Verification items for the finished model (mm, model axes). A direction names the side the tool comes from. Give positions to 0.01 mm unless a question says otherwise; leave off trailing zeros. Order: outer loops, then holes, each group sorted by start corner. A loop starts at its lowest first (then second) coordinate and runs counter-clockwise, first axis right, second up. Notation, with made-up numbers: (5, 61) -> (48, 61) arc R13 cw to (48, 79) -> close; hole circle Ø2 at (16, 29.25). An arc over 180 degrees is marked (long way). Return JSON: item names as keys, results as strings. Group by question number.
(1) Tool access check on faces 1 (the face through (73.74, 16.07, -5.06)), 2 (the face through (9.648, 0.359, 16.406)). Record the directions out of +Z, -Z, +X, -X, +Y, -Y that give a thin tool (end or side, any length) a straight path to the whole face; none if there is none.
(2) Depth check by flat-ended pin: pin 1 Ø6 at (x, y) = (115.5, 7.5) entering from -Z; pin 2 Ø1 at (x, y) = (53, 12) entering from +Z; pin 3 Ø1.5 at (x, z) = (51.5, 8) entering from -Y. Enter the tip coordinate at first touch or a pass-through.
(3) Cross-section at B-B on x = 69. Enter the section's corners in (y, z).
(4) Release check for a two-part mould opening along X. For faces 3 (the face through (75.81, 15.28, -4.81)), 4 (the face through (-0.25, -1.953, -14.877)) record: pulls with the +X half, pulls with the -X half, needs draft (parallel to the pull), parting line crosses it, or undercut.
(5) Cross-section at A-A on z = 0. Enter the section's corners in (x, y).
(6) Thickness scan on line 1 along Y through (x, z) = (79, 0); line 2 along Z through (x, y) = (149.85, 0). Record the ranges inside material, lowest first.
from build123d import *

# Parameters (mm, degrees)
SKETCH2_R          = 1.1938
CUT_EXTRUDE1_DEPTH = 16.84655


with BuildPart() as part:
    # Sketch1 → Revolve1 (revolve)
    with BuildSketch(Plane.XY):
        with BuildLine():
            Line((-0.882617928, 15.379667928), (-0.508, 15.00505))
            Line((-0.508, 15.00505), (0, 15.00505))
            Line((0, 15.00505), (1.016, 16.02105))
            Line((1.016, 16.02105), (148.5392, 16.02105))
            Line((148.5392, 16.02105), (149.5552, 15.00505))
            Line((149.5552, 15.00505), (150.0632, 15.00505))
            Line((150.0632, 15.00505), (150.437817928, 15.379667928))
            ThreePointArc((150.437817928, 15.379667928), (150.475015367, 15.46947049), (150.437817928, 15.559273051))
            Line((150.437817928, 15.559273051), (149.44812049, 16.54897049))
            ThreePointArc((149.44812049, 16.54897049), (149.118506367, 16.769211605), (148.7297, 16.84655))
            Line((148.7297, 16.84655), (0.8255, 16.84655))
            ThreePointArc((0.8255, 16.84655), (0.436693633, 16.769211605), (0.10707951, 16.54897049))
            Line((0.10707951, 16.54897049), (-0.882617928, 15.559273051))
            ThreePointArc((-0.882617928, 15.559273051), (-0.919815367, 15.46947049), (-0.882617928, 15.379667928))
        make_face()
    revolve(axis=Axis((149.5552, 0, 0), (-1, 0, 0)))

    # Sketch2 → Cut-Extrude1 (cut)
    with BuildSketch(Plane.XY):
        with Locations((8.509, 0)):
            Circle(SKETCH2_R)
    extrude(amount=CUT_EXTRUDE1_DEPTH, mode=Mode.SUBTRACT)


solid = part.part
Verdict:
{
 "1": {"face 1": "+X, -X", "face 2": "+Z"},
 "2": {"pin 1": "z = -16.23", "pin 2": "z = 12.31", "pin 3": "y = -15.21"},
 "3": {"outline": "circle Ø33.69 at (0, 0); hole circle Ø32.04 at (0, 0)"},
 "4": {"face 3": "undercut", "face 4": "needs draft"},
 "5": {"outline": "(-0.88, -15.56) -> (0.11, -16.55) arc R1.02 ccw to (0.83, -16.85) -> (148.73, -16.85) arc R1.02 ccw to (149.45, -16.55) -> (150.44, -15.56) arc R0.13 ccw to (150.44, -15.38) -> (150.06, -15.01) -> (149.56, -15.01) -> (148.54, -16.02) -> (1.02, -16.02) -> (0, -15.01) -> (-0.51, -15.01) -> (-0.88, -15.38) arc R0.13 ccw to start; (-0.88, 15.38) -> (-0.51, 15.01) -> (0, 15.01) -> (1.02, 16.02) -> (148.54, 16.02) -> (149.56, 15.01) -> (150.06, 15.01) -> (150.44, 15.38) arc R0.13 ccw to (150.44, 15.56) -> (149.45, 16.55) arc R1.02 ccw to (148.73, 16.85) -> (0.83, 16.85) arc R1.02 ccw to (0.11, 16.55) -> (-0.88, 15.56) arc R0.13 ccw to start"},
 "6": {"line 1": "-16.85 to -16.02, 16.02 to 16.85", "line 2": "-16.15 to -15.01, 15.01 to 16.15"}
}
